Source: three-view drawing plus pictorial views. Frame: mm from the lowest corner of the part. A direction names the side the tool comes from. Coordinates: 2 decimals unless noted, no trailing zeros. Order: outer loops, then holes, each group sorted by start corner. A loop starts at its lowest first (then second) coordinate and runs counter-clockwise, first axis right, second up. Notation, with made-up numbers: M 22.5,69.5 L 35.5,69.5 A27 ccw 35.5,100.5 Z; hole C 70.25,6 d6. An arc over 180 degrees is marked long. Use CSV: the item, a comma, the result in double quotes. Start each with the question number.
Q1. First-contact query: P1, Ø5, axis at y = 18.5, z = 23, coming from the +X side; P2, Ø1.5, axis at x = 85, z = 8.5, coming from the +Y side; P3, Ø22, axis at x = 122, z = 10.5, coming from the +Y side; P4, Ø12, axis at y = 14.5, z = 8.5, coming from the +X side. Flat tips, straight axial feed; report the tip coordinate or a pass-through.
Q2. Mould query, pull axis Y, two halves, no side actions, for the marked faces 5, 6 and 7. Classes: +Y half, -Y half, draft (parallel to the pull), parting line (faces both ways), or undercut.
Q3. Section query C-C, the plane z = 45.5. Output: boundary loops of the cut face in (x, y), and give its area (3 significant figures).
Q4. Ray query, probe 1 along X at (y, z) = (39, 41); probe 2 along Y at (x, z) = (60.5, 16.5); probe 3 along X at (y, z) = (47, 9). Return the intervals inside material, ascending.
Q5. Section query B-B, the plane y = 40. Output: boundary loops of the cut face in (x, z).
Q6. Section query A-A, the plane x = 80. Output: boundary loops of the cut face in (y, z), and give its area (3 significant figures).
Q7. Section query D-D, the plane x = 48. Output: boundary loops of the cut face in (y, z), and give its area (3 significant figures).
Q8. Access query for the marked faces 1, 2, 3 and 4. Directions: +Z, -Z, +X, -X, +Y, -Y. A direction counts if a zero-diameter tool reaches every point of the face in a straight line with its end or side. Return the directions, or none.
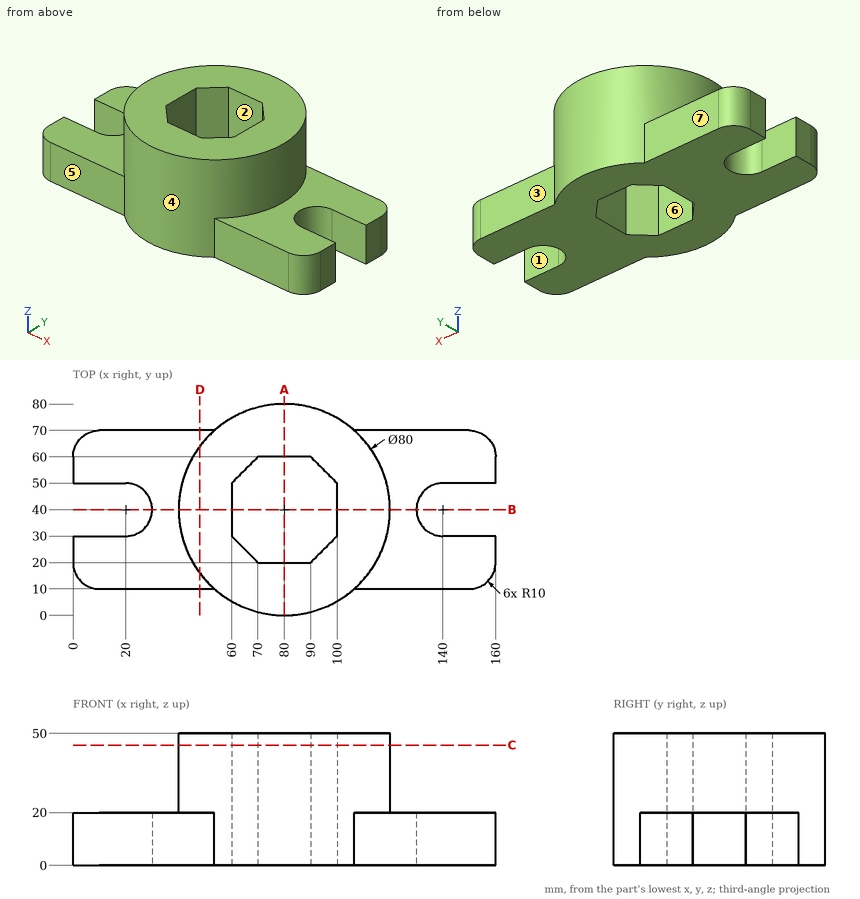
Responses:
1,P1,"stops at x = 115.2"
1,P2,"stops at y = 79.77"
1,P3,"stops at y = 70"
1,P4,"stops at x = 160"
2,face 5,"-Y half"
2,face 6,"undercut"
2,face 7,"+Y half"
3,outline,"C 80,40 d80; hole M 60,30 L 70,20 L 90,20 L 100,30 L 100,50 L 90,60 L 70,60 L 60,50 Z"
3,area,"3,630 mm²"
4,probe 1,"x = 40.01 to 60, 100 to 119.99"
4,probe 2,"y = 5.08 to 29.5, 50.5 to 74.92"
4,probe 3,"x = 27.14 to 60, 100 to 132.86"
5,outline,"M 30,0 L 60,0 L 60,50 L 40,50 L 40,20 L 30,20 Z; M 100,0 L 130,0 L 130,20 L 120,20 L 120,50 L 100,50 Z"
6,outline,"M 0,0 L 20,0 L 20,50 L 0,50 Z; M 60,0 L 80,0 L 80,50 L 60,50 Z"
6,area,"2,000 mm²"
7,outline,"M 10,0 L 70,0 L 70,20 L 64,20 L 64,50 L 16,50 L 16,20 L 10,20 Z"
7,area,"2,640 mm²"
8,face 1,"+Z, -Z, +X"
8,face 2,"+Z, -Z"
8,face 3,"+Z, -Z, +X, +Y"
8,face 4,"+Z"
